CAD build for the part. Positions are in the model's coordinates, mm. Face numbers are marked on the shaded views. A direction names the side the tool comes from. Coordinates: 2 decimals unless noted, no trailing zeros. Loops run counter-clockwise (first coordinate to the right, second up) from the corner with the lowest first, then second, coordinate; pieces in that order, holes last. Notation, with made-up numbers: (5, 31.25) - (59, 31.25) arc R4 cw to (59, 37.25) - close; hole circle Ø5 at (0, 56.25). An arc over 180 degrees is marked (long way). Put each result on its own line as item: value.
```python
from build123d import *

# Parameters (mm, degrees)
ESQUISSE1_R                  = 11
ESQUISSE1_R_2                = 7
EXTRUSION1_DEPTH             = 63
CHANFREIN1_SIZE              = 1
ENL_V_MAT_EXTRU_1_DEPTH      = 8.5
R_P_TITION_CIRCULAIRE1_COUNT = 8
SYM_TRIE1_COPY_1_DEPTH       = 8.5
SYM_TRIE1_COPY_2_DEPTH       = 8.5
SYM_TRIE1_COPY_3_DEPTH       = 8.5
SYM_TRIE1_COPY_4_DEPTH       = 8.5
SYM_TRIE1_COPY_5_DEPTH       = 8.5
SYM_TRIE1_COPY_6_DEPTH       = 8.5
SYM_TRIE1_COPY_7_DEPTH       = 8.5


with BuildPart() as part:
    # Esquisse1 → Extrusion1 (new body, symmetric)
    with BuildSketch(Plane(origin=(0, 0, 0), x_dir=(1, 0, 0), z_dir=(0, 1, 0))):
        with Locations(Location((0, 0, 0), (0, 0, 270))):  # turned: the seam where the file's is
            Circle(ESQUISSE1_R)
        with Locations(Location((0, 0, 0), (0, 0, 270))):  # turned: the seam where the file's is
            Circle(ESQUISSE1_R_2, mode=Mode.SUBTRACT)
    extrude(amount=EXTRUSION1_DEPTH, both=True)

    # Esquisse3 → Enlèvement de matière-Révolution2 (revolve, cut)
    with BuildSketch(Plane.XY, mode=Mode.PRIVATE) as enl_vement_de_mati_re_r_volution2_sk:
        Polygon((10.7, 63), (10.7, 53), (10.75, 53), (11, 38.677509592), (11, 63), align=None)
        Polygon((11, -63), (10.7, -63), (10.7, -53), (10.75, -53), (11, -38.677509592), align=None)
    revolve(enl_vement_de_mati_re_r_volution2_sk.sketch.rotate(Axis((0, 68.024691358, 0), (0, -1, 0)), 90), axis=Axis((0, 68.024691358, 0), (0, -1, 0)), mode=Mode.SUBTRACT)  # turned: the seam where the file's is

    # Chanfrein1
    chanfrein1_edges = [part.edges().sort_by_distance(p)[0] for p in [
        (0, 63, -10.7),
        (0, -63, -10.7),
    ]]
    chamfer(chanfrein1_edges, length=CHANFREIN1_SIZE)

    # Esquisse4 → Enlèv. mat.-Extru.1 (cut)
    with BuildSketch(Plane(origin=(0, 63, 0), x_dir=(-1, 0, 0), z_dir=(0, 1, 0))):
        with BuildLine():
            Line((1.5, -10.594338111), (1.5, -8.366600265))
            ThreePointArc((1.5, -8.366600265), (0, -8.5), (-1.5, -8.366600265))
            Line((-1.5, -8.366600265), (-1.5, -10.594338111))
            ThreePointArc((-1.5, -10.594338111), (0, -10.7), (1.5, -10.594338111))
        make_face()
    enl_v_mat_extru_1 = extrude(amount=-ENL_V_MAT_EXTRU_1_DEPTH, mode=Mode.SUBTRACT)

    # Répétition circulaire1: Enlèv. mat.-Extru.1 ×8 about axis
    r_p_tition_circulaire1_axis = Axis((0, 0, 0), (0, 1, 0))
    for i in range(1, R_P_TITION_CIRCULAIRE1_COUNT):
        add(enl_v_mat_extru_1.rotate(r_p_tition_circulaire1_axis, i * 360 / R_P_TITION_CIRCULAIRE1_COUNT), mode=Mode.SUBTRACT)

    # Symétrie1: Enlèv. mat.-Extru.1 across plane
    add(enl_v_mat_extru_1.mirror(Plane.ZX), mode=Mode.SUBTRACT)

    # Symétrie1 copy 1 sketch → Symétrie1 copy 1 (cut)
    with BuildSketch(Plane(origin=(0, -63, 0), x_dir=(-0.707106781, 0, 0.707106781), z_dir=(0, -1, 0))):
        with BuildLine():
            Line((1.5, 10.594338111), (1.5, 8.366600265))
            ThreePointArc((1.5, 8.366600265), (0, 8.5), (-1.5, 8.366600265))
            Line((-1.5, 8.366600265), (-1.5, 10.594338111))
            ThreePointArc((-1.5, 10.594338111), (0, 10.7), (1.5, 10.594338111))
        make_face()
    extrude(amount=-SYM_TRIE1_COPY_1_DEPTH, mode=Mode.SUBTRACT)

    # Symétrie1 copy 2 sketch → Symétrie1 copy 2 (cut)
    with BuildSketch(Plane(origin=(0, -63, 0), x_dir=(0, 0, 1), z_dir=(0, -1, 0))):
        with BuildLine():
            Line((1.5, 10.594338111), (1.5, 8.366600265))
            ThreePointArc((1.5, 8.366600265), (0, 8.5), (-1.5, 8.366600265))
            Line((-1.5, 8.366600265), (-1.5, 10.594338111))
            ThreePointArc((-1.5, 10.594338111), (0, 10.7), (1.5, 10.594338111))
        make_face()
    extrude(amount=-SYM_TRIE1_COPY_2_DEPTH, mode=Mode.SUBTRACT)

    # Symétrie1 copy 3 sketch → Symétrie1 copy 3 (cut)
    with BuildSketch(Plane(origin=(0, -63, 0), x_dir=(0.707106781, 0, 0.707106781), z_dir=(0, -1, 0))):
        with BuildLine():
            Line((1.5, 10.594338111), (1.5, 8.366600265))
            ThreePointArc((1.5, 8.366600265), (0, 8.5), (-1.5, 8.366600265))
            Line((-1.5, 8.366600265), (-1.5, 10.594338111))
            ThreePointArc((-1.5, 10.594338111), (0, 10.7), (1.5, 10.594338111))
        make_face()
    extrude(amount=-SYM_TRIE1_COPY_3_DEPTH, mode=Mode.SUBTRACT)

    # Symétrie1 copy 4 sketch → Symétrie1 copy 4 (cut)
    with BuildSketch(Plane.XZ.offset(63)):
        with BuildLine():
            Line((1.5, 10.594338111), (1.5, 8.366600265))
            ThreePointArc((1.5, 8.366600265), (0, 8.5), (-1.5, 8.366600265))
            Line((-1.5, 8.366600265), (-1.5, 10.594338111))
            ThreePointArc((-1.5, 10.594338111), (0, 10.7), (1.5, 10.594338111))
        make_face()
    extrude(amount=-SYM_TRIE1_COPY_4_DEPTH, mode=Mode.SUBTRACT)

    # Symétrie1 copy 5 sketch → Symétrie1 copy 5 (cut)
    with BuildSketch(Plane(origin=(0, -63, 0), x_dir=(0.707106781, 0, -0.707106781), z_dir=(0, -1, 0))):
        with BuildLine():
            Line((1.5, 10.594338111), (1.5, 8.366600265))
            ThreePointArc((1.5, 8.366600265), (0, 8.5), (-1.5, 8.366600265))
            Line((-1.5, 8.366600265), (-1.5, 10.594338111))
            ThreePointArc((-1.5, 10.594338111), (0, 10.7), (1.5, 10.594338111))
        make_face()
    extrude(amount=-SYM_TRIE1_COPY_5_DEPTH, mode=Mode.SUBTRACT)

    # Symétrie1 copy 6 sketch → Symétrie1 copy 6 (cut)
    with BuildSketch(Plane(origin=(0, -63, 0), x_dir=(0, 0, -1), z_dir=(0, -1, 0))):
        with BuildLine():
            Line((1.5, 10.594338111), (1.5, 8.366600265))
            ThreePointArc((1.5, 8.366600265), (0, 8.5), (-1.5, 8.366600265))
            Line((-1.5, 8.366600265), (-1.5, 10.594338111))
            ThreePointArc((-1.5, 10.594338111), (0, 10.7), (1.5, 10.594338111))
        make_face()
    extrude(amount=-SYM_TRIE1_COPY_6_DEPTH, mode=Mode.SUBTRACT)

    # Symétrie1 copy 7 sketch → Symétrie1 copy 7 (cut)
    with BuildSketch(Plane(origin=(0, -63, 0), x_dir=(-0.707106781, 0, -0.707106781), z_dir=(0, -1, 0))):
        with BuildLine():
            Line((1.5, 10.594338111), (1.5, 8.366600265))
            ThreePointArc((1.5, 8.366600265), (0, 8.5), (-1.5, 8.366600265))
            Line((-1.5, 8.366600265), (-1.5, 10.594338111))
            ThreePointArc((-1.5, 10.594338111), (0, 10.7), (1.5, 10.594338111))
        make_face()
    extrude(amount=-SYM_TRIE1_COPY_7_DEPTH, mode=Mode.SUBTRACT)


solid = part.part
```
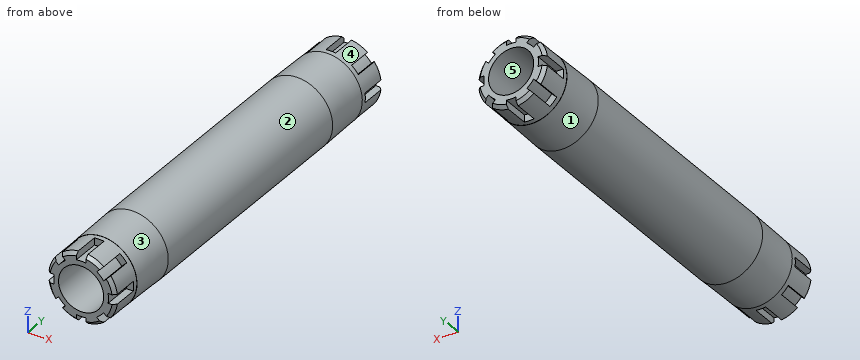
Q1. Tool access for the marked faces 1, 2 and 3: list every direction of +Z, -Z, +X, -X, +Y, -Y with a clear straight run to the whole face (end or side of a thin tool).
Determined:
face 1: +Y
face 2: +Y, -Y
face 3: -Y
Q2. Mould opens along X. For the marked faces 4 and 5 say: +X half, -X half, draft (parallel to the pull), parting line (faces both ways), or undercut.
Determined:
face 4: parting line
face 5: undercut
Q3. Wall check: L1, parallel to X at y = -20, z = 0; L2, parallel to Z at x = -5.75, y = 56; L3, parallel to Z at x = -1, y = -6.5. Give the ranges that are in metal, low to high. Write a range as from..to.
Determined:
L1: -11..-7, 7..11
L2: -9.02..-7.87, -6.26..-3.99, 3.99..6.26, 7.87..9.02
L3: -10.95..-6.93, 6.93..10.95
Q4. Slice it at A-A, the plane y = -20. Give the cut face in (x, z), then the cut area to 3 significant figures.
Determined:
outline: circle Ø22 at (0, 0); hole circle Ø14 at (0, 0)
area: 226 mm2
Q5. Pin check, flat tips, straight feed: pin 1 Ø2.5 at (x, y) = (-10, -60.5) entering from +Z; pin 2 Ø5 at (y, z) = (-15.5, 6.5) entering from -X; pin 3 Ø5 at (y, z) = (-39, -6) entering from +X. Stop position of each tip, or through.
Determined:
pin 1: z = 6.16
pin 2: x = -10.25
pin 3: x = 10.42
